Job drawing, mm, ordinate dimensions from the low corner. One solid piece. Give positions to 0.01 mm unless a question says otherwise; leave off trailing zeros. Order: outer loops, then holes, each group sorted by start corner. A loop starts at its lowest first (then second) coordinate and runs counter-clockwise, first axis right, second up. Notation, with made-up numbers: (-11, 57.25) -> (3, 57.25) arc R15 ccw to (3, 72.25) -> close; hole circle Ø11 at (-23.5, 86). An arc over 180 degrees is marked (long way). Write item = value, one per line. Start each with the question number.
(1) Probe line 1 along X through (y, z) = (1.2, 33); line 2 along Z through (x, y) = (78.5, 0.5); line 3 along Z through (x, y) = (107, 0.75) (1 decimal). List the from-to ranges inside material, lowest first. Write a range as from..to.
(2) Saw through at A-A, the plane y = 1.1. List the corners of the cut face in (x, z).
(3) Saw through at C-C, the plane x = 113.5. List the corners of the cut face in (y, z) (1 decimal).
(4) Saw through at B-B, the plane x = 42.5. List the corners of the cut face in (y, z) (1 decimal), then the cut area to 3 significant figures.
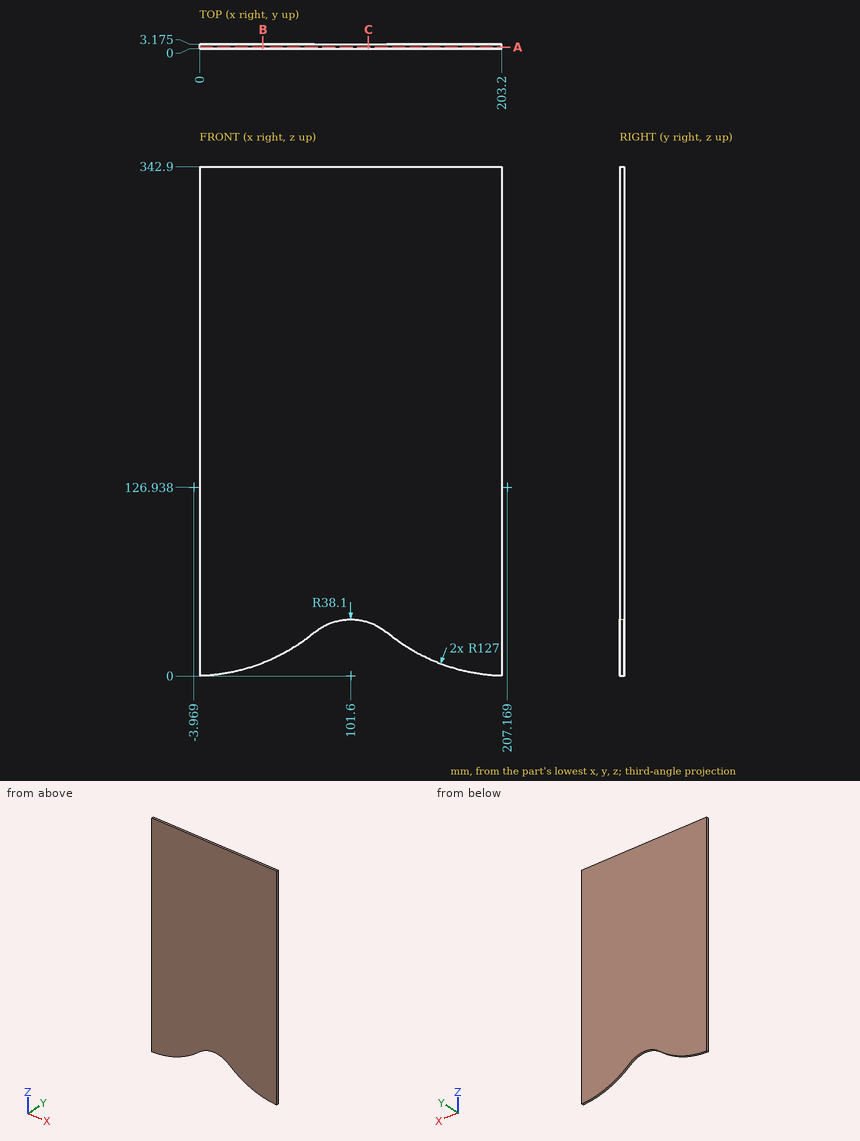
Results list:
q1.line_1 = 0..82.56, 120.64..203.2
q1.line_2 = 30.3..342.9
q1.line_3 = 37.7..342.9
q2.outline = (0, 0) arc R127 ccw to (77.24, 29.29) arc R38.1 cw to (125.96, 29.29) arc R127 ccw to (203.2, 0) -> (203.2, 342.9) -> (0, 342.9) -> close
q3.outline = (0, 36.2) -> (3.2, 36.2) -> (3.2, 342.9) -> (0, 342.9) -> close
q4.outline = (0, 8.7) -> (3.2, 8.7) -> (3.2, 342.9) -> (0, 342.9) -> close
q4.area = 1,060 mm^2
